Design review of the part built by this model. Coordinates are the model's own, in mm. Face numbers are marked on the shaded views. Give positions to 0.01 mm unless a question says otherwise; leave off trailing zeros. Write each loop counter-clockwise with the first axis right and the second up, starting at its lowest first coordinate (ties: lowest second). Pieces come first, ordered by that corner, then holes. Notation, with made-up numbers: (32.25, -31) -> (62.25, -31) arc R18 cw to (62.25, 4) -> close; hole circle Ø5 at (-29.5, 73). An arc over 180 degrees is marked (long way). Write each question's results on one line, items separated by ' | '. Start each with the question number.
(1) Mouldability with a two-part tool opening along Y and no side actions: class the marked faces 1 and 2 as released by +Y, released by -Y, zero draft, split by the parting line, or undercut.
(2) Take a section at A-A (y = 0). State the section outline as (x, z) points, plus the area to 3 significant figures.
(3) To check wall thickness, follow probe 1 along Y at (x, z) = (0, 53); probe 2 along Z at (x, y) = (-3.5, 12.5); probe 3 along Y at (x, z) = (10.5, 52.5). State the ranges of each line that lie inside material, in increasing order.
(4) Take a section at B-B (x = 0). State the section outline as (y, z) points.
(5) Take a section at C-C (z = 74). State the section outline as (x, y) points, plus the area to 3 significant figures.
(6) Take a section at D-D (y = 12.5). State the section outline as (x, z) points.
(7) Clearance check with flat-ended pins moving along their axes: pin 1 (0.9 mm diameter, centred on x = 10.5, y = 5.5, fed in from +Z); pin 2 (2 mm diameter, centred on x = -8.5, z = 47.5, fed in from +Y); pin 3 (2 mm diameter, centred on x = -2.5, z = 42, fed in from -Y). State where each tip first meets the part, or that it passes through.
from build123d import *

# Parameters (mm, degrees)
SKETCH1_R           = 18
BOSS_EXTRUDE1_DEPTH = 60
SKETCH2_R           = 2.5
BOSS_EXTRUDE2_DEPTH = 20
SKETCH3_R           = 1.5
CUT_EXTRUDE1_DEPTH  = 10


with BuildPart() as part:
    # Sketch1 → Boss-Extrude1 (new body)
    with BuildSketch(Plane.XY):
        Circle(SKETCH1_R)
    extrude(amount=BOSS_EXTRUDE1_DEPTH)

    # Sketch2 → Boss-Extrude2 (add)
    with BuildSketch(Plane.XY.offset(60)):
        Circle(SKETCH2_R)
    extrude(amount=BOSS_EXTRUDE2_DEPTH)

    # Sketch3 → Cut-Extrude1 (cut)
    with BuildSketch(Plane.XY.offset(60)):
        with Locations((0, 12.5)):
            Circle(SKETCH3_R)
        with Locations((10.825317547, 6.25)):
            Circle(SKETCH3_R)
        with Locations((10.825317547, -6.25)):
            Circle(SKETCH3_R)
        with Locations((0, -12.5)):
            Circle(SKETCH3_R)
        with Locations((-10.825317547, -6.25)):
            Circle(SKETCH3_R)
        with Locations((-10.825317547, 6.25)):
            Circle(SKETCH3_R)
    extrude(amount=-CUT_EXTRUDE1_DEPTH, mode=Mode.SUBTRACT)


solid = part.part
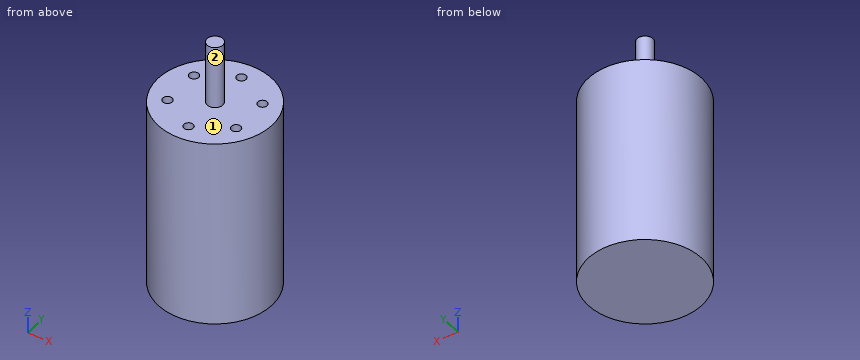
Report:
1) face 1: zero draft | face 2: split by the parting line
2) outline: (-18, 0) -> (18, 0) -> (18, 60) -> (2.5, 60) -> (2.5, 80) -> (-2.5, 80) -> (-2.5, 60) -> (-18, 60) -> close | area: 2,260 mm2
3) probe 1: -18 to -14, -11 to 11, 14 to 18 | probe 2: 0 to 60 | probe 3: -14.62 to -7.71, -4.79 to 4.79, 7.71 to 14.62
4) outline: (-18, 0) -> (18, 0) -> (18, 60) -> (14, 60) -> (14, 50) -> (11, 50) -> (11, 60) -> (2.5, 60) -> (2.5, 80) -> (-2.5, 80) -> (-2.5, 60) -> (-11, 60) -> (-11, 50) -> (-14, 50) -> (-14, 60) -> (-18, 60) -> close
5) outline: circle Ø5 at (0, 0) | area: 19.6 mm2
6) outline: (-12.95, 0) -> (12.95, 0) -> (12.95, 60) -> (1.5, 60) -> (1.5, 50) -> (-1.5, 50) -> (-1.5, 60) -> (-12.95, 60) -> close
7) pin 1: z = 50 | pin 2: y = 16.36 | pin 3: y = -17.94
